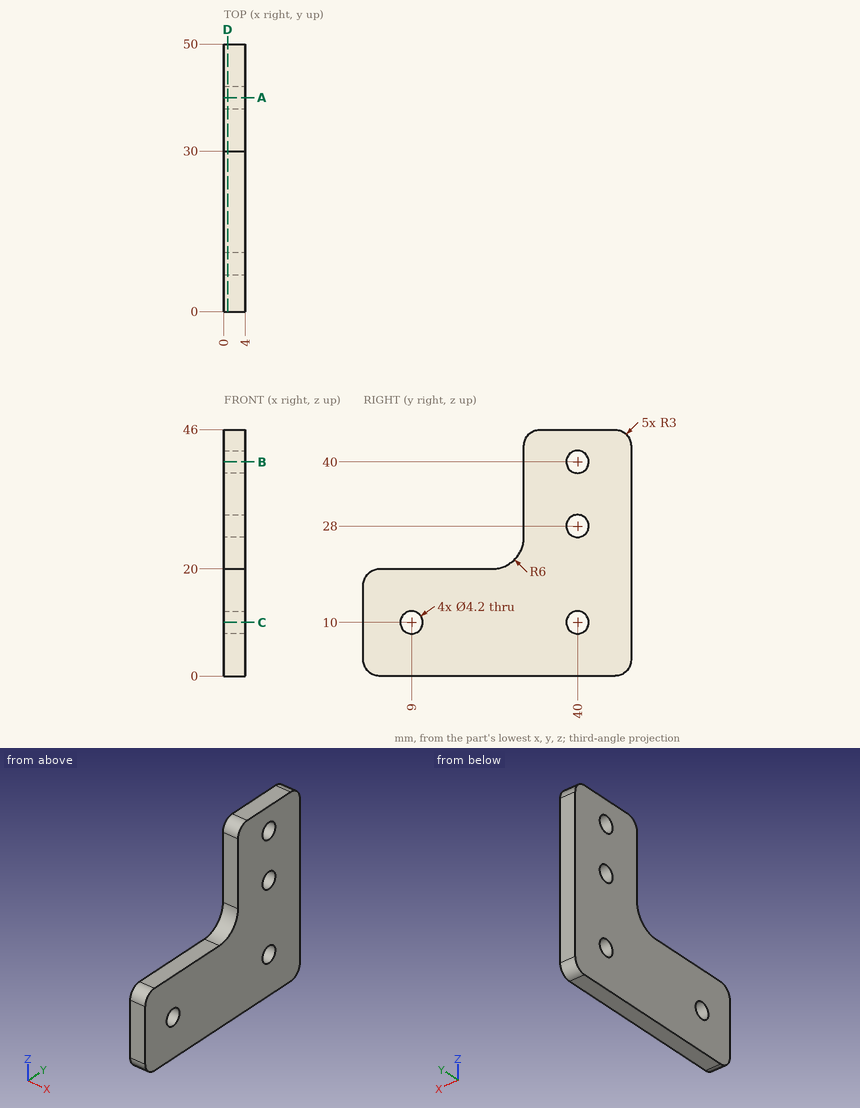
Source: three-view drawing plus pictorial views. Frame: mm from the lowest corner of the part. Round coordinates to 2 decimals unless told otherwise and drop trailing zeros. Write each loop counter-clockwise with the first axis right and the second up, starting at its lowest first coordinate (ties: lowest second). Pieces come first, ordered by that corner, then holes. Notation, with made-up numbers: (-33.75, 44.5) -> (-12.75, 44.5) arc R23 ccw to (-12.75, 52.5) -> close; hole circle Ø4 at (-21, -22). An arc over 180 degrees is marked (long way). Return JSON: item names as keys, results as strings.
Q1. First-contact query: pin 1 Ø2.5 at (y, z) = (40, 10) entering from -X; pin 2 Ø2 at (x, z) = (2.5, 32.5) entering from -Y; pin 3 Ø1.5 at (x, y) = (1, 7.5) entering from +Z. Flat tips, straight axial feed; report the tip coordinate or a pass-through.
From the geometry:
{"pin 1": "through", "pin 2": "y = 30", "pin 3": "z = 20"}
Q2. Section A-A on y = 40. Return the cut outline in (x, z), and give its area (3 significant figures).
From the geometry:
{"outline": "(0, 0) -> (4, 0) -> (4, 7.9) -> (0, 7.9) -> close; (0, 12.1) -> (4, 12.1) -> (4, 25.9) -> (0, 25.9) -> close; (0, 30.1) -> (4, 30.1) -> (4, 37.9) -> (0, 37.9) -> close; (0, 42.1) -> (4, 42.1) -> (4, 46) -> (0, 46) -> close", "area": "134 mm2"}
Q3. Section B-B on z = 40. Return the cut outline in (x, y), and give its area (3 significant figures).
From the geometry:
{"outline": "(0, 30) -> (4, 30) -> (4, 37.9) -> (0, 37.9) -> close; (0, 42.1) -> (4, 42.1) -> (4, 50) -> (0, 50) -> close", "area": "63.2 mm2"}
Q4. Section C-C on z = 10. Return the cut outline in (x, y).
From the geometry:
{"outline": "(0, 0) -> (4, 0) -> (4, 6.9) -> (0, 6.9) -> close; (0, 11.1) -> (4, 11.1) -> (4, 37.9) -> (0, 37.9) -> close; (0, 42.1) -> (4, 42.1) -> (4, 50) -> (0, 50) -> close"}
Q5. Ray query, line 1 (Y direction, x = 1.2, z = 10); line 2 (Y direction, x = 1.5, z = 28); line 3 (Y direction, x = 3.8, z = 27). Return the intervals inside material, ascending.
From the geometry:
{"line 1": "0 to 6.9, 11.1 to 37.9, 42.1 to 50", "line 2": "30 to 37.9, 42.1 to 50", "line 3": "30 to 38.15, 41.85 to 50"}
Q6. Section D-D on x = 0.7. Return the cut outline in (y, z).
From the geometry:
{"outline": "(0, 3) arc R3 ccw to (3, 0) -> (47, 0) arc R3 ccw to (50, 3) -> (50, 43) arc R3 ccw to (47, 46) -> (33, 46) arc R3 ccw to (30, 43) -> (30, 26) arc R6 cw to (24, 20) -> (3, 20) arc R3 ccw to (0, 17) -> close; hole circle Ø4.2 at (9, 10); hole circle Ø4.2 at (40, 10); hole circle Ø4.2 at (40, 28); hole circle Ø4.2 at (40, 40)"}
